```python
from build123d import *

# Parameters (mm, degrees)
EXTRUDE_1_DEPTH     = 10
SKETCH_2_R          = 1
CUT_EXTRUDE_1_DEPTH = 39.925698452
SKETCH_3_R          = 2.5
CUT_EXTRUDE_2_DEPTH = 5
CUT_EXTRUDE_START   = -31.4
SKETCH_3_2_R        = 2.5
CUT_EXTRUDE_3_DEPTH = 5
FILLET_1_R          = 3
FILLET_2_R          = 0.2


with BuildPart() as part:
    # 스케치1 → 보스-돌출1 (new body)
    with BuildSketch(Plane.XY):
        Polygon((18.2, 9.5), (-18.2, 9.5), (-18.2, -9.5), (-13.5, -9.5), (-13.5, -6.5), (-7.5, -6.5), (-7.5, 4.5), (7.5, 4.5), (7.5, -6.5), (13.5, -6.5), (13.5, -9.5), (18.2, -9.5), align=None)
    extrude(amount=EXTRUDE_1_DEPTH)

    # 스케치2 → 컷-돌출1 (cut, through all)
    with BuildSketch(Plane(origin=(18.2, 0, 0), x_dir=(0, 0, -1), z_dir=(1, 0, 0))):
        with Locations(Location((-5, -1, 0), (0, 0, 90))):
            Circle(SKETCH_2_R)
    extrude(amount=-CUT_EXTRUDE_1_DEPTH, mode=Mode.SUBTRACT)

    # 스케치3 → 컷-돌출2 (cut)
    with BuildSketch(Plane(origin=(18.2, 0, 0), x_dir=(0, 0, -1), z_dir=(1, 0, 0))):
        with Locations(Location((-5, -1, 0), (0, 0, 90))):
            Circle(SKETCH_3_R)
    extrude(amount=-CUT_EXTRUDE_2_DEPTH, mode=Mode.SUBTRACT)

    # 스케치3<2> → 컷-돌출3 (cut)
    with BuildSketch(Plane(origin=(18.2, 0, 0), x_dir=(0, 0, -1), z_dir=(1, 0, 0)).offset(CUT_EXTRUDE_START)):
        with Locations(Location((-5, -1, 0), (0, 0, 90))):
            Circle(SKETCH_3_2_R)
    extrude(amount=-CUT_EXTRUDE_3_DEPTH, mode=Mode.SUBTRACT)

    # 필렛1
    fillet_1_edges = [part.edges().sort_by_distance(p)[0] for p in [
        (-18.2, -9.5, 5),
        (-18.2, 9.5, 5),
        (18.2, 9.5, 5),
        (18.2, -9.5, 5),
    ]]
    fillet(fillet_1_edges, radius=FILLET_1_R)

    # 필렛2
    fillet_2_edges = [part.edges().sort_by_distance(p)[0] for p in [
        (14.35, -9.5, 10),
        (10.5, -6.5, 0),
        (7.5, -1, 0),
        (0, 4.5, 0),
        (-7.5, -1, 0),
        (-10.5, -6.5, 0),
        (-13.5, -8, 0),
        (14.35, -9.5, 0),
        (13.5, -8, 0),
        (-13.5, -8, 10),
        (-10.5, -6.5, 10),
        (-7.5, -1, 10),
        (0, 4.5, 10),
        (7.5, -1, 10),
        (-14.35, -9.5, 0),
        (-14.35, -9.5, 10),
        (10.5, -6.5, 10),
        (-18.2, 0, 0),
        (13.5, -8, 10),
        (0, 9.5, 0),
        (18.2, 0, 0),
        (17.321320344, 8.621320344, 0),
        (-17.321320344, 8.621320344, 0),
        (17.321320344, -8.621320344, 0),
        (-17.321320344, -8.621320344, 0),
        (-18.2, 0, 10),
        (18.2, 0, 10),
        (0, 9.5, 10),
        (17.321320344, 8.621320344, 10),
        (-17.321320344, 8.621320344, 10),
        (17.321320344, -8.621320344, 10),
        (-17.321320344, -8.621320344, 10),
    ]]
    fillet(fillet_2_edges, radius=FILLET_2_R)


solid = part.part
```
CAD build for the part. Positions are in the model's coordinates, mm. A direction names the side the tool comes from. Give positions to 0.01 mm unless a question says otherwise; leave off trailing zeros. Order: outer loops, then holes, each group sorted by start corner. A loop starts at its lowest first (then second) coordinate and runs counter-clockwise, first axis right, second up.
(1) Saw through at A-A, the plane z = 5. State how many separate pieces and enclosed holes the cut face has, then the cut area to 3 significant figures.
(2) Saw through at C-C, the plane x = 10. Give the cut face in (y, z), then the cut area to 3 significant figures.
(3) Saw through at D-D, the plane y = 3.25. Give the cut face in (x, z), then the cut area to 3 significant figures.
(4) Flat gauge pins, fed straight in: pin 1 (1.5 mm diameter, centred on x = 7, z = 7.5, fed in from -Y); pin 2 (4.5 mm diameter, centred on y = -1, z = 5, fed in from -X); pin 3 (3.5 mm diameter, centred on y = -8.5, z = 6, fed in from -X); pin 4 (4 mm diameter, centred on y = -0.5, z = 5.5, fed in from +X). Where does each tip first touch, or does it go through?
(5) Mould opens along Z. For faces 6 (the flat face through (13.2, 0, 4)), 7 (the flat face through (0, 9.5, 5)), 8 (the flat face through (0, 6, 0)) say: released by +Z, released by -Z, zero draft, split by the parting line, or undercut.
(6) Tool access for faces 1 (the cylindrical face through (-10, -1, 6)), 2 (the flat face through (-13.2, 0, 4)), 3 (the flat face through (-13.5, -8, 5)), 4 (the cylindrical face through (15.74, -1.33, 7.48)), 5 (the cylindrical face through (-17.3, 8.64, 5.07)): list every direction of +Z, -Z, +X, -X, +Y, -Y with a clear straight run to the whole face (end or side of a thin tool).
(7) Drill centre lines: L1, parallel to Z at x = -9.85, y = -1; L2, parallel to Z at x = 17, y = -1; L3, parallel to X at y = -3.5, z = 3.5. Where is each one in solid material? Low to high.
Results found:
1. separate pieces: 3
1. enclosed holes: 0
1. area: 365 mm2
2. outline: (-6.5, 0.2) arc R0.2 ccw to (-6.3, 0) - (9.3, 0) arc R0.2 ccw to (9.5, 0.2) - (9.5, 9.8) arc R0.2 ccw to (9.3, 10) - (-6.3, 10) arc R0.2 ccw to (-6.5, 9.8) - close; hole circle Ø2 at (-1, 5)
2. area: 157 mm2
3. outline: (-18.2, 0.2) arc R0.2 ccw to (-18, 0) - (-7.7, 0) arc R0.2 ccw to (-7.5, 0.2) - (-7.5, 9.8) arc R0.2 ccw to (-7.7, 10) - (-18, 10) arc R0.2 ccw to (-18.2, 9.8) - close; (7.5, 0.2) arc R0.2 ccw to (7.7, 0) - (18, 0) arc R0.2 ccw to (18.2, 0.2) - (18.2, 9.8) arc R0.2 ccw to (18, 10) - (7.7, 10) arc R0.2 ccw to (7.5, 9.8) - close
3. area: 214 mm2
4. pin 1: stops at y = -6.5
4. pin 2: stops at x = -13.2
4. pin 3: stops at x = -18.19
4. pin 4: stops at x = 18.2
5. face 6: undercut
5. face 7: zero draft
5. face 8: released by -Z
6. face 1: +X, -X
6. face 2: -X
6. face 3: +Z, -Z, -Y
6. face 4: +X
6. face 5: +Z, -Z, -X, +Y
7. L1: z = 0 to 4, 6 to 10
7. L2: z = 0 to 2.5, 7.5 to 10
7. L3: x = -18.2 to -7.5, 7.5 to 18.2
